Here's how the part is built. I have some questions about the finished solid (model axes, mm). A direction names the side the tool comes from. Coordinates: 2 decimals unless noted, no trailing zeros. Loops run counter-clockwise (first coordinate to the right, second up) from the corner with the lowest first, then second, coordinate; pieces in that order, holes last.
from build123d import *

# Parameters (mm, degrees)
SKETCH1_W               = 50
SKETCH1_H               = 31.5
BOSS_EXTRUDE1_DEPTH     = 23
CUT_EXTRUDE1_DEPTH      = 20
CUT_EXTRUDE2_DEPTH      = 57.769820327
CUT_EXTRUDE2_DEPTH_BACK = 57.769820327
SKETCH3_R               = 0.8


with BuildPart() as part:
    # Sketch1 → Boss-Extrude1 (new body)
    with BuildSketch(Plane(origin=(0, 0, 0), x_dir=(1, 0, 0), z_dir=(0, 1, 0))):
        with Locations((25, 15.75)):
            Rectangle(SKETCH1_W, SKETCH1_H)
    extrude(amount=BOSS_EXTRUDE1_DEPTH)

    # Sketch2 → Cut-Extrude1 (cut)
    with BuildSketch(Plane(origin=(0, 23, 0), x_dir=(1, 0, 0), z_dir=(0, 1, 0))):
        Polygon((41.25, 28.5), (8.75, 28.5), (8.75, 25.5), (6.75, 25.5), (6.75, 6), (8.75, 6), (8.75, 3), (41.25, 3), (41.25, 8.2), (42.4, 8.2), (42.4, 23.3), (41.25, 23.3), align=None)
    extrude(amount=-CUT_EXTRUDE1_DEPTH, mode=Mode.SUBTRACT)

    # Sketch3 → Cut-Extrude2 (cut, two sides: drawn at the far end of the back side and taken through both)
    with BuildSketch(Plane.ZY.offset(-41.25).offset(-CUT_EXTRUDE2_DEPTH_BACK)):
        with Locations(Location((-26.55, 9, 0), (0, 0, 180))):
            Circle(SKETCH3_R)
        with Locations(Location((-6.05, 9, 0), (0, 0, 273.583321698))):
            Circle(SKETCH3_R)
    extrude(amount=CUT_EXTRUDE2_DEPTH + CUT_EXTRUDE2_DEPTH_BACK, mode=Mode.SUBTRACT)


solid = part.part
Q1. For faces 4 (the flat face through (8, 16, -6)), 5 (the flat face through (25, 11, -31.5)), which set-ups out of +Z, -Z, +X, -X, +Y, -Y let a thin tool reach every point of the face, with its end or its side?
Q2. Will these pins go through, and if not, where does the flat tip stop? P1, Ø12, axis at x = 31, y = 5, coming from the +Z side; P2, Ø1.3, axis at y = 9, z = -6.05, coming from the -X side; P3, Ø13, axis at x = 23.5, z = -12, coming from the +Y side.
Q3. Suppose I cut it at B-B on y = 9. State how many separate pieces and enclosed holes the cut face has, and give its area (3 significant figures).
Q4. Suppose I cut it at A-A on z = -26.55. Write out the boundary of the cut face in (x, y), and give its area (3 significant figures).
Q5. We'd pull the mould along Y, two halves only. Please class faces 1 (the flat face through (25, 0, -16)), 2 (the cylindrical face through (4.44, 8.61, -5.35)), 3 (the flat face through (0, 11, -16)): pulls with the +Y half, pulls with the -Y half, needs draft (parallel to the pull), parting line crosses it, or undercut.
Q6. Please list where these lines run through material, in increasing order: probe 1 along X at (y, z) = (15, -15); probe 2 along Y at (x, z) = (3.25, -6.05); probe 3 along Z at (x, y) = (7, 19).
Q7. Suppose I cut it at D-D on x = 17.5. Write out the boundary of the cut face in (y, z).
Q8. Suppose I cut it at C-C on y = 17. Write out the boundary of the cut face in (x, z), and give its area (3 significant figures).
Check values:
1. face 4: +Y
1. face 5: -Z, +X, -X, +Y, -Y
2. P1: stops at z = 0
2. P2: passes through
2. P3: stops at y = 3
3. separate pieces: 4
3. enclosed holes: 0
3. area: 636 mm2
4. outline: (0, 0) - (50, 0) - (50, 8.2) - (41.25, 8.2) - (41.25, 3) - (8.75, 3) - (8.75, 8.2) - (0, 8.2) - close; (0, 9.8) - (8.75, 9.8) - (8.75, 23) - (0, 23) - close; (41.25, 9.8) - (50, 9.8) - (50, 23) - (41.25, 23) - close
4. area: 472 mm2
5. face 1: pulls with the -Y half
5. face 2: undercut
5. face 3: needs draft
6. probe 1: x = 0 to 6.75, 42.4 to 50
6. probe 2: y = 0 to 8.2, 9.8 to 23
6. probe 3: z = -31.5 to -25.5, -6 to 0
7. outline: (0, -31.5) - (23, -31.5) - (23, -28.5) - (3, -28.5) - (3, -3) - (23, -3) - (23, 0) - (0, 0) - close
8. outline: (0, -31.5) - (50, -31.5) - (50, 0) - (0, 0) - close; hole (6.75, -25.5) - (8.75, -25.5) - (8.75, -28.5) - (41.25, -28.5) - (41.25, -23.3) - (42.4, -23.3) - (42.4, -8.2) - (41.25, -8.2) - (41.25, -3) - (8.75, -3) - (8.75, -6) - (6.75, -6) - close
8. area: 690 mm2
